Check sheet for the modelled part. Datum: model origin and axes. Units: mm. A direction names the side the tool comes from. Coordinates: 2 decimals unless noted, no trailing zeros. Write each loop counter-clockwise with the first axis right and the second up, starting at its lowest first coordinate (ties: lowest second). Pieces come first, ordered by that corner, then holes. Notation, with made-up numbers: M 27,84 L 66,84 A11 cw 66,94 Z; hole C 40,-21.75 d10. An arc over 180 degrees is marked long. Answer as CSV lines item,"result".
from build123d import *

# Parameters (mm, degrees)
EXTRUDE_1_DEPTH     = 3
CUT_EXTRUDE_1_DEPTH = 10
SKETCH_3_R          = 3
CUT_EXTRUDE_2_DEPTH = 1.5
SKETCH_4_R          = 1.425
CUT_EXTRUDE_3_DEPTH = 2
CUT_EXTRUDE_4_DEPTH = 0.2
CUT_EXTRUDE_START   = -10
CUT_EXTRUDE_5_DEPTH = 10


with BuildPart() as part:
    # Эскиз1 → Бобышка-Вытянуть1 (new body)
    with BuildSketch(Plane.XY):
        with BuildLine():
            Line((-52.5, -90), (52.5, -90))
            ThreePointArc((52.5, -90), (59.571067812, -87.071067812), (62.5, -80))
            Line((62.5, -80), (62.5, 80))
            ThreePointArc((62.5, 80), (59.571067812, 87.071067812), (52.5, 90))
            Line((52.5, 90), (-52.5, 90))
            ThreePointArc((-52.5, 90), (-59.571067812, 87.071067812), (-62.5, 80))
            Line((-62.5, 80), (-62.5, -80))
            ThreePointArc((-62.5, -80), (-59.571067812, -87.071067812), (-52.5, -90))
        make_face()
    extrude(amount=EXTRUDE_1_DEPTH)

    # Эскиз2 → Вырез-Вытянуть1 (cut)
    with BuildSketch(Plane(origin=(0, 0, 0), x_dir=(-1, 0, 0), z_dir=(0, 0, -1))):
        with BuildLine():
            Line((-36.25, -44), (-36.25, -46))
            ThreePointArc((-36.25, -46), (-35.298097039, -48.298097039), (-33, -49.25))
            Line((-33, -49.25), (-32.75, -49.25))
            ThreePointArc((-32.75, -49.25), (-18.607864376, -55.107864376), (-12.75, -69.25))
            Line((-12.75, -69.25), (-12.75, -79.25))
            ThreePointArc((-12.75, -79.25), (-12.164213562, -80.664213562), (-10.75, -81.25))
            Line((-10.75, -81.25), (10.75, -81.25))
            ThreePointArc((10.75, -81.25), (12.164213562, -80.664213562), (12.75, -79.25))
            Line((12.75, -79.25), (12.75, -69.25))
            ThreePointArc((12.75, -69.25), (18.607864376, -55.107864376), (32.75, -49.25))
            Line((32.75, -49.25), (33, -49.25))
            ThreePointArc((33, -49.25), (35.298097039, -48.298097039), (36.25, -46))
            Line((36.25, -46), (36.25, -44))
            ThreePointArc((36.25, -44), (35.298097039, -41.701902961), (33, -40.75))
            Line((33, -40.75), (-33, -40.75))
            ThreePointArc((-33, -40.75), (-35.298097039, -41.701902961), (-36.25, -44))
        make_face()
    extrude(amount=-CUT_EXTRUDE_1_DEPTH, mode=Mode.SUBTRACT)

    # Эскиз3 → Вырез-Вытянуть2 (cut)
    with BuildSketch(Plane.XY.offset(3)):
        with Locations((0, 88)):
            Circle(SKETCH_3_R)
        with Locations((60.5, 0)):
            Circle(SKETCH_3_R)
        with Locations((0, -88)):
            Circle(SKETCH_3_R)
        with Locations((-60.5, 0)):
            Circle(SKETCH_3_R)
    extrude(amount=-CUT_EXTRUDE_2_DEPTH, mode=Mode.SUBTRACT)

    # Эскиз4 → Вырез-Вытянуть3 (cut)
    with BuildSketch(Plane.XY.offset(1.5)):
        with Locations((0, 88)):
            Circle(SKETCH_4_R)
        with Locations((60.5, 0)):
            Circle(SKETCH_4_R)
        with Locations((0, -88)):
            Circle(SKETCH_4_R)
        with Locations((-60.5, 0)):
            Circle(SKETCH_4_R)
    extrude(amount=-CUT_EXTRUDE_3_DEPTH, mode=Mode.SUBTRACT)

    # Эскиз5 → Вырез-Вытянуть4 (cut)
    with BuildSketch(Plane.XY.offset(3)):
        with BuildLine():
            Line((-10.25, -0.09106889), (-10.25, -16.21851864))
            ThreePointArc((-10.25, -16.21851864), (-9.664213562, -17.632732202), (-8.25, -18.21851864))
            Line((-8.25, -18.21851864), (-7.25, -18.21851864))
            ThreePointArc((-7.25, -18.21851864), (-5.835786438, -17.632732202), (-5.25, -16.21851864))
            Line((-5.25, -16.21851864), (-5.25, -7.46851864))
            ThreePointArc((-5.25, -7.46851864), (-4.883883476, -6.584635164), (-4, -6.21851864))
            Line((-4, -6.21851864), (4, -6.21851864))
            ThreePointArc((4, -6.21851864), (4.883883476, -6.584635164), (5.25, -7.46851864))
            Line((5.25, -7.46851864), (5.25, -16.21851864))
            ThreePointArc((5.25, -16.21851864), (5.835786438, -17.632732202), (7.25, -18.21851864))
            Line((7.25, -18.21851864), (8.25, -18.21851864))
            ThreePointArc((8.25, -18.21851864), (9.664213562, -17.632732202), (10.25, -16.21851864))
            Line((10.25, -16.21851864), (10.25, -0.09106889))
            ThreePointArc((10.25, -0.09106889), (10.971727173, 1.041815844), (12.303484512, 0.866486664))
            Line((12.303484512, 0.866486664), (15.917557024, -2.166080248))
            ThreePointArc((15.917557024, -2.166080248), (16.829986215, -2.453768066), (17.67859709, -2.012009206))
            Line((17.67859709, -2.012009206), (19.022071027, -0.410919315))
            ThreePointArc((19.022071027, -0.410919315), (19.309758846, 0.501509876), (18.867999985, 1.350120751))
            Line((18.867999985, 1.350120751), (10.947043439, 7.996592468))
            ThreePointArc((10.947043439, 7.996592468), (10.195124773, 8.430712912), (9.340074414, 8.58148136))
            Line((9.340074414, 8.58148136), (7.25, 8.58148136))
            ThreePointArc((7.25, 8.58148136), (5.835786438, 7.995694922), (5.25, 6.58148136))
            Line((5.25, 6.58148136), (5.25, -0.16851864))
            ThreePointArc((5.25, -0.16851864), (4.883883476, -1.052402116), (4, -1.41851864))
            Line((4, -1.41851864), (-4, -1.41851864))
            ThreePointArc((-4, -1.41851864), (-4.883883476, -1.052402116), (-5.25, -0.16851864))
            Line((-5.25, -0.16851864), (-5.25, 6.58148136))
            ThreePointArc((-5.25, 6.58148136), (-5.835786438, 7.995694922), (-7.25, 8.58148136))
            Line((-7.25, 8.58148136), (-9.340074414, 8.58148136))
            ThreePointArc((-9.340074414, 8.58148136), (-10.195124773, 8.430712912), (-10.947043439, 7.996592468))
            Line((-10.947043439, 7.996592468), (-18.867999985, 1.350120751))
            ThreePointArc((-18.867999985, 1.350120751), (-19.309758846, 0.501509876), (-19.022071027, -0.410919315))
            Line((-19.022071027, -0.410919315), (-17.67859709, -2.012009206))
            ThreePointArc((-17.67859709, -2.012009206), (-16.829986215, -2.453768066), (-15.917557024, -2.166080248))
            Line((-15.917557024, -2.166080248), (-12.303484512, 0.866486664))
            ThreePointArc((-12.303484512, 0.866486664), (-10.971727173, 1.041815844), (-10.25, -0.09106889))
        make_face()
        with BuildLine():
            Line((0, 14.858517807), (-4.979473915, 19.036792532))
            ThreePointArc((-4.979473915, 19.036792532), (-6.074388944, 19.382017915), (-7.092721994, 18.851907282))
            Line((-7.092721994, 18.851907282), (-8.483871936, 17.193999341))
            ThreePointArc((-8.483871936, 17.193999341), (-8.829097318, 16.099084312), (-8.298986686, 15.080751262))
            Line((-8.298986686, 15.080751262), (-1.285575219, 9.195800287))
            ThreePointArc((-1.285575219, 9.195800287), (0, 8.727889173), (1.285575219, 9.195800287))
            Line((1.285575219, 9.195800287), (8.298986686, 15.080751262))
            ThreePointArc((8.298986686, 15.080751262), (8.829097318, 16.099084312), (8.483871936, 17.193999341))
            Line((8.483871936, 17.193999341), (7.092721994, 18.851907282))
            ThreePointArc((7.092721994, 18.851907282), (6.074388944, 19.382017915), (4.979473915, 19.036792532))
            Line((4.979473915, 19.036792532), (0, 14.858517807))
        make_face()
    extrude(amount=-CUT_EXTRUDE_4_DEPTH, mode=Mode.SUBTRACT)

    # Эскиз8 → Вырез-Вытянуть5 (cut)
    with BuildSketch(Plane.XY.offset(3).offset(CUT_EXTRUDE_START)):
        with BuildLine():
            Line((-52.5, 90), (-42.5, 90))
            Line((-42.5, 90), (-42.5, 86))
            Line((-42.5, 86), (-55.5, 86))
            ThreePointArc((-55.5, 86), (-57.621320344, 85.121320344), (-58.5, 83))
            Line((-58.5, 83), (-58.5, 70))
            Line((-58.5, 70), (-62.5, 70))
            Line((-62.5, 70), (-62.5, 80))
            ThreePointArc((-62.5, 80), (-59.571067812, 87.071067812), (-52.5, 90))
        make_face()
        with BuildLine():
            Line((62.5, 70), (62.5, 80))
            ThreePointArc((62.5, 80), (59.571067812, 87.071067812), (52.5, 90))
            Line((52.5, 90), (42.5, 90))
            Line((42.5, 90), (42.5, 86))
            Line((42.5, 86), (55.5, 86))
            ThreePointArc((55.5, 86), (57.621320344, 85.121320344), (58.5, 83))
            Line((58.5, 83), (58.5, 70))
            Line((58.5, 70), (62.5, 70))
        make_face()
        with BuildLine():
            Line((52.5, -90), (42.5, -90))
            Line((42.5, -90), (42.5, -86))
            Line((42.5, -86), (55.5, -86))
            ThreePointArc((55.5, -86), (57.621320344, -85.121320344), (58.5, -83))
            Line((58.5, -83), (58.5, -70))
            Line((58.5, -70), (62.5, -70))
            Line((62.5, -70), (62.5, -80))
            ThreePointArc((62.5, -80), (59.571067812, -87.071067812), (52.5, -90))
        make_face()
        with BuildLine():
            Line((-62.5, -70), (-62.5, -80))
            ThreePointArc((-62.5, -80), (-59.571067812, -87.071067812), (-52.5, -90))
            Line((-52.5, -90), (-42.5, -90))
            Line((-42.5, -90), (-42.5, -86))
            Line((-42.5, -86), (-55.5, -86))
            ThreePointArc((-55.5, -86), (-57.621320344, -85.121320344), (-58.5, -83))
            Line((-58.5, -83), (-58.5, -70))
            Line((-58.5, -70), (-62.5, -70))
        make_face()
    extrude(amount=CUT_EXTRUDE_5_DEPTH, mode=Mode.SUBTRACT)


solid = part.part
1) Thickness scan on line 1 along Y through (x, z) = (0, 0.45) (3 decimals); line 2 along X through (y, z) = (-78, 0.4); line 3 along X through (y, z) = (88, 2.2). Record the ranges inside material, lowest first.
Answer key:
line 1,"y = -90 to -89.425, -86.575 to -81.25, -40.75 to 86.575, 89.425 to 90"
line 2,"x = -58.5 to -12.75, 12.75 to 58.5"
line 3,"x = -42.5 to -3, 3 to 42.5"
2) Section check B-B, the plane x = 48. Record the boundary of the cut face in (y, z).
Answer key:
outline,"M -86,0 L 86,0 L 86,3 L -86,3 Z"
3) Depth check by flat-ended pin: P1, Ø1.5, axis at x = 61, y = 1.5, coming from the +Z side; P2, Ø1.5, axis at x = -52, z = 2, coming from the +Y side; P3, Ø1.5, axis at x = -61, z = 1.5, coming from the -Y side. Enter the tip coordinate at first touch or a pass-through.
Answer key:
P1,"stops at z = 1.5"
P2,"stops at y = 86"
P3,"stops at y = -70"
4) Mould release check, pull along Y, two halves, no side actions. Record for faces 4 (the face through (0, 85, 2)), 5 (the face through (-1, 1, 0)), 6 (the face through (0, 86, 1.5)): pulls with the +Y half, pulls with the -Y half, needs draft (parallel to the pull), parting line crosses it, or undercut.
Answer key:
face 4,"undercut"
face 5,"needs draft"
face 6,"undercut"
5) Tool access check on faces 1 (the face through (-1, 1, 3)), 2 (the face through (18.764, -54.953, 1.479)), 3 (the face through (0, -86, 1.5)). Record the directions out of +Z, -Z, +X, -X, +Y, -Y that give a thin tool (end or side, any length) a straight path to the whole face; none if there is none.
Answer key:
face 1,"+Z, +X, -X, +Y, -Y"
face 2,"+Z, -Z"
face 3,"+Z"
6) Section check A-A, the plane x = -25. Record the boundary of the cut face in (y, z).
Answer key:
outline,"M -90,0 L -50.81,0 L -50.81,3 L -90,3 Z; M -40.75,0 L 90,0 L 90,3 L -40.75,3 Z"
7) Section check C-C, the plane z = 0.45. Give the number of separate pieces and of enclosed holes in the cut face, plus the area to 3 significant figures.
Answer key:
separate pieces,"1"
enclosed holes,"5"
area,"20,300 mm2"
